Build history of the part. All positions in model axes, mm. A direction names the side the tool comes from. Round coordinates to 2 decimals unless told otherwise and drop trailing zeros. Write each loop counter-clockwise with the first axis right and the second up, starting at its lowest first coordinate (ties: lowest second). Pieces come first, ordered by that corner, then holes. Notation, with made-up numbers: (-12, 88) - (32, 88) arc R16 ccw to (32, 99) - close; hole circle Ø9 at (28.25, 23). An arc over 180 degrees is marked (long way). Write each question's results on one line, items separated by ' | '.
Autodesk Inventor part; units mm, degrees
ref_plane "Work Plane1" through (29, 0, 0) normal (0, -1, 0) x (1, 0, 0)
ref_plane "YZ Plane" through (0, 0, 0) normal (1, 0, 0) x (0, 1, 0)
ref_plane "XZ Plane" through (0, 0, 0) normal (0, 1, 0) x (-1, 0, 0)
sketch "Sketch1" plane through (0, 0, 0) normal (0, 0, 1) x (1, 0, 0)
  line L0 (0.3333, 0) -> (16, 0)
  line L1 (16, 0) -> (16, 2)
  line L2 (16, 2) -> (2.1, 2)
  line L3 (2.1, 2) -> (1.6705, 2)
  line L4 (1.6705, 2) -> (0, 2)
  line L5 (0, 2) -> (0, 3.5)
  line L6 (0, 3.5) -> (-2.8, 3.5)
  line L7 (-2.8, 3.5) -> (-2.8, 1.4434)
  line L8 (-2.8, 1.4434) -> (-0.5, 1.4434)
  line L9 (-0.5, 1.4434) -> (0.3333, 0)
  line L10 (-6.56, 0) -> (19.76, 0)
  line L11 (0, -0.7) -> (0, 4.2)
  line L12 (2.1, 2) -> (0, 2) construction
  dimension "d1" = 13.9
  dimension "d2" = 0.4295
  dimension "d3" = 2.8
  dimension "d4" = 2.3
  dimension "d5" = 60
  dimension "d6" = 4
  dimension "d7" = 4
  dimension "d8" = 2.8868
  dimension "d9" = 7
  dimension "d26" = 16
revolve "Body" add sketch "Sketch1" angle 360 about axis through (0.3333, 0, 0) along (1, 0, 0) contours L9 L11 L4 L3 L2 L1 L0 | L9 L8 L7 L6 L5 L11
sketch "Sketch2" plane through (-2.8, 0, 0) normal (-1, 0, 0) x (0, 0, 1)
  circle A0 centre (0, 0) radius 1.4434
  line L0 (0, -4.9) -> (0, 4.9)
  line L1 (-4.9, 0) -> (4.9, 0)
  line L2 (1.4434, 0) -> (0.7217, -1.25)
  line L3 (0.7217, -1.25) -> (-0.7217, -1.25)
  line L4 (-0.7217, -1.25) -> (-1.4434, 0)
  line L5 (-1.4434, 0) -> (-0.7217, 1.25)
  line L6 (-0.7217, 1.25) -> (0.7217, 1.25)
  line L7 (0.7217, 1.25) -> (1.4434, 0)
extrude "Slot" add sketch "Sketch2" against normal up to next contours L7 A0 | A0 L2 | L6 L0 A0 | A0 L0 L3 | L0 L6 A0 | A0 L3 L0 | L4 A0 | A0 L5
fillet "Fillet1" radius 0.4 1 edges at (-2.8, -3.5, 0)
thread "Thread"
chamfer "Chamfer1" distance 0.4294 distance2 0.4294 1 edges at (16, -2, 0) measured on face at (16, 0.527, -0.2661)
ref_plane "Work Plane1" through (29, 0, 0) normal (0, -1, 0) x (1, 0, 0)
fillet "Fillet2" radius 0.1 1 edges at (0, -2, 0)
equation "\"d1\" = GEL"
equation "\"d3\" = KOH"
equation "\"d4\" = INTI"
equation "\"d6\" = GD"
equation "\"d7\" = BDM"
equation "\"d8\" = 1.1547 * SW"
equation "\"d9\" = KOD"
equation "\"d26\" = NLG"
equation "\"d30\" = R"
equation "\"d17\" = RR"
equation "\"d13\" = GEL"
equation "\"d15\" = -0.5 * SPD + 0.5 * GD"
equation "\"d16\" = GUL"
equation "\"GD\" = NND"
equation "\"NLG\" = 16"
equation "\"GEL\" = 13.9"
equation "\"KOD\" = 7"
equation "\"KOH\" = 2.8"
equation "\"INTI\" = 2.3"
equation "\"GAL\" = 0.61345 * PTC"
equation "\"GUL\" = 0.61345 * PTC"
equation "\"BDM\" = NND"
equation "\"SW\" = 2.5"
equation "\"RR\" = 0.4"
equation "\"SPD\" = NND - 1.2269 * PTC"
equation "\"R\" = 0.1"
equation "\"TOA\" = 30deg"
equation "\"GD1\" = THREADDIA - 1.2269 * PTC"
equation "\"THREADDIA\" = 4"
equation "\"FAWI\" = 45deg"
equation "\"ANG\" = 120deg"
equation "\"PTC\" = 0.7"
equation "\"NND\" = 4"
equation "\"E0\" = 1.155 * SW"
properties part number "DIN 7984 - M4 x 16" material "Steel, Mild"
(1) Drill centre lines: probe 1 along X at (y, z) = (2.5, 0.25); probe 2 along Z at (x, y) = (9.25, 0.5); probe 3 along Y at (x, z) = (5.75, -1.5). Where is each one in solid material? Low to high. Write a range as [from, to].
Worked answers:
probe 1: x = [-2.8, 0] | probe 2: z = [-1.94, 1.94] | probe 3: y = [-1.32, 1.32]
(2) Tool access for faces 5 (the flat face through (-2, 1.25, 0)), 6 (the flat face through (-2.8, -0.6, 1.3)), 7 (the flat face through (0, 2, -2)): list every direction of +Z, -Z, +X, -X, +Y, -Y with a clear straight run to the whole face (end or side of a thin tool).
Worked answers:
face 5: -X | face 6: +Z, -Z, -X, +Y, -Y | face 7: +X
(3) Two-plate mould, pull along Z, no slides. Class faces 1 (the flat face through (-1.611, 0.616, -1.088)), 2 (the cylindrical face through (8, 0, 2)), 3 (the conical face through (0.28, 0.09, -0.03)), 4 (the flat face through (16, 0, 0)): released by +Z, released by -Z, zero draft, split by the parting line, or undercut.
Worked answers:
face 1: undercut | face 2: split by the parting line | face 3: undercut | face 4: zero draft
(4) Slice it at B-B, the plane x = 2. Write the cut outline in (y, z).
Worked answers:
outline: circle Ø4 at (0, 0)
(5) Slice it at A-A, the plane x = -1. Write the cut outline in (y, z).
Worked answers:
outline: circle Ø7 at (0, 0); hole (-1.25, -0.72) - (0, -1.44) - (1.25, -0.72) - (1.25, 0.72) - (0, 1.44) - (-1.25, 0.72) - close
